```python
from build123d import *

# Parameters (mm, degrees)
SKETCH013_W = 1.38
SKETCH013_H = 6


with BuildPart() as part:
    # AdditivePipe004: sweep along a path in Sketch014
    with BuildLine(Plane.XY) as additivepipe004_path:
        Line((12.38, -10), (12.38, 0))
        ThreePointArc((12.38, 0), (6.88, 5.5), (1.38, 0))
        Line((1.38, 0), (1.38, -10))
    # Sketch013 → AdditivePipe004 (sweep)
    with BuildSketch(Plane.XZ):
        with Locations((0.69, 3)):
            Rectangle(SKETCH013_W, SKETCH013_H)
    sweep(path=additivepipe004_path.line)


solid = part.part
```
Here's how the part is built. I have some questions about the finished solid (model axes, mm). A direction names the side the tool comes from. Coordinates: 2 decimals unless noted, no trailing zeros. Order: outer loops, then holes, each group sorted by start corner. A loop starts at its lowest first (then second) coordinate and runs counter-clockwise, first axis right, second up.
Item 1: If we section it at C-C, the plane x = 6.88: List the corners of the cut face in (y, z) for me.
Response values:
outline: (5.5, 0) - (6.88, 0) - (6.88, 6) - (5.5, 6) - close
Item 2: If we section it at A-A, the plane y = -2: List the corners of the cut face in (x, z) for me.
Response values:
outline: (0, 0) - (1.38, 0) - (1.38, 6) - (0, 6) - close; (12.38, 0) - (13.76, 0) - (13.76, 6) - (12.38, 6) - close
Item 3: Thinking about a two-plate mould opening in X: for faces 3 (the face through (13.76, -5, 3)), 4 (the face through (1, 0, 6)), 5 (the face through (1.38, -5, 3)), which applies, pulls with the +X half, pulls with the -X half, needs draft (parallel to the pull), parting line crosses it, or undercut?
Response values:
face 3: pulls with the +X half
face 4: needs draft
face 5: undercut
Item 4: Which directions (+Z, -Z, +X, -X, +Y, -Y) give clear straight access to the entire face, cutting with the end or side of a thin tool? Please do faces 1 (the face through (13, -10, 3)), 2 (the face through (12.38, -5, 3)).
Response values:
face 1: +Z, -Z, +X, -X, -Y
face 2: +Z, -Z, -Y
Item 5: I'm going to push a flat-ended pin straight in: pin 1 Ø1 at (x, y) = (7.5, 3) entering from +Z. Where does the tip first touch, or does it pass through?
Response values:
pin 1: passes through
Item 6: If we section it at D-D, the plane y = 1.75: List the corners of the cut face in (x, z) for me, then the cut area to 3 significant figures.
Response values:
outline: (0.23, 0) - (1.67, 0) - (1.67, 6) - (0.23, 6) - close; (12.09, 0) - (13.53, 0) - (13.53, 6) - (12.09, 6) - close
area: 17.3 mm2
Item 7: If we section it at B-B, the plane z = 0.75: List the corners of the cut face in (x, y) for me.
Response values:
outline: (0, -10) - (1.38, -10) - (1.38, 0) arc R5.5 cw to (12.38, 0) - (12.38, -10) - (13.76, -10) - (13.76, 0) arc R6.88 ccw to (0, 0) - close
Item 8: I need wall thicknesses on probe 1 along X at (y, z) = (-6, 1.3); probe 2 along X at (y, z) = (2.25, 4.75); probe 3 along Y at (x, z) = (2, 0.3). Which ranges of each line are inside material? Lowest first, please.
Response values:
probe 1: x = 0 to 1.38, 12.38 to 13.76
probe 2: x = 0.38 to 1.86, 11.9 to 13.38
probe 3: y = 2.54 to 4.85
